Can you work these out from the model? Positions are in its coordinate system, mm. A direction names the side the tool comes from. Give positions to 0.01 mm unless a question says otherwise; leave off trailing zeros. Write each loop counter-clockwise with the first axis right and the second up, starting at its lowest first coordinate (ties: lowest second). Pieces come first, ordered by that corner, then holes. Notation, with made-up numbers: (48.5, 17.25) -> (67.5, 17.25) arc R28 cw to (67.5, 54.25) -> close; hole circle Ø8 at (79.5, 2.5). An arc over 180 degrees is marked (long way). Answer as CSV lines item,"result". Start each with the question number.
1. If we section it at D-D on z = -27: Write out the boundary of the cut face in (x, y).
2. I need wall thicknesses on line 1 (X direction, y = 17, z = -23); line 2 (Y direction, x = 25.5, z = 0); line 3 (Y direction, x = 39, z = 0). Which ranges of each line are inside material? Lowest first, please. Write a range as [from, to].
3. I'm going to push flat-ended pins straight in: P1, Ø21.5, axis at y = 0, z = 0, coming from the -X side; P2, Ø4, axis at y = -1, z = 11.5, coming from the -X side; P3, Ø6, axis at y = -28, z = -3.5, coming from the +X side; P4, Ø12, axis at y = -27, z = 19, coming from the -X side. Where does each tip first touch, or does it pass through?
4. If we mould it in two halves opening along X, with no side actions, what happens to faces 1 (the face through (-45.491, 16, 1)), 2 (the face through (-46.03, -23.81, -22.88)), 3 (the face through (20.707, -9, -4))? For each: pulls with the +X half, pulls with the -X half, needs draft (parallel to the pull), parting line crosses it, or undercut.
5. If we section it at C-C on x = 3: Write out the boundary of the cut face in (y, z).
6. On a 3-axis mill with a long thin cutter (end or side, diameter ignored), from which of +Z, -Z, +X, -X, +Y, -Y can I reach the whole of each face in a straight line? I mean faces 4 (the face through (-16.35, 7.19, 9.37)), 5 (the face through (45.491, -1, 16)), 6 (the face through (49.212, 9.35, -7.47)), 7 (the face through (46.045, -12.053, -11.283)), 8 (the face through (37.91, 7.19, 9.37)). Say none if no direction works.
```python
from build123d import *

# Parameters (mm, degrees)
CUT_EXTRUDE1_DEPTH      = 111.87459973
CUT_EXTRUDE1_DEPTH_BACK = 111.87459973


with BuildPart() as part:
    # Sketch2 → Revolve1 (revolve)
    with BuildSketch(Plane.XY, mode=Mode.PRIVATE) as revolve1_sk:
        Polygon((-52.3875, 11.811), (-52.3875, 12.7), (-46.5836, 12.7), (-46.5836, 36.83), (-45.4914, 36.83), (-45.4914, 12.7), (45.4914, 12.7), (45.4914, 36.83), (46.5836, 36.83), (46.5836, 12.7), (49.2125, 12.7), (49.2125, 11.811), (26.91765, 11.811), (26.91765, 9.36625), (20.70735, 9.36625), (20.70735, 11.811), align=None)
    revolve(revolve1_sk.sketch.rotate(Axis((0, 0, 0), (-1, 0, 0)), 90), axis=Axis((0, 0, 0), (-1, 0, 0)))

    # Sketch3 → Cut-Extrude1 (cut, two sides: drawn at the far end of the back side and taken through both)
    with BuildSketch(Plane.ZY.offset(-45.4914).offset(-CUT_EXTRUDE1_DEPTH_BACK)):
        with BuildLine():
            Line((-18.112952688, -5.32652278), (-29.140106204, -8.569306297))
            ThreePointArc((-29.140106204, -8.569306297), (-30.702095808, -9.883795088), (-30.792130213, -11.923301428))
            ThreePointArc((-30.792130213, -11.923301428), (-22.728159534, -23.953103435), (-10.291997319, -31.375072768))
            ThreePointArc((-10.291997319, -31.375072768), (-8.264508496, -31.180706004), (-7.031658144, -29.559419671))
            Line((-7.031658144, -29.559419671), (-4.327850892, -18.394165222))
            ThreePointArc((-4.327850892, -18.394165222), (-4.548475673, -16.613982469), (-5.890298237, -15.423504358))
            ThreePointArc((-5.890298237, -15.423504358), (-11.349323888, -11.990535738), (-15.076837789, -6.728228762))
            ThreePointArc((-15.076837789, -6.728228762), (-16.331679174, -5.457246069), (-18.112952688, -5.32652278))
        make_face()
    extrude(amount=CUT_EXTRUDE1_DEPTH + CUT_EXTRUDE1_DEPTH_BACK, mode=Mode.SUBTRACT)


solid = part.part
```
Computed values:
1,outline,"(-46.58, -25.05) -> (-45.49, -25.05) -> (-45.49, -19.01) -> (-46.58, -19.01) -> close; (-46.58, -7.94) -> (-45.49, -7.94) -> (-45.49, 25.05) -> (-46.58, 25.05) -> close; (45.49, -25.05) -> (46.58, -25.05) -> (46.58, -19.01) -> (45.49, -19.01) -> close; (45.49, -7.94) -> (46.58, -7.94) -> (46.58, 25.05) -> (45.49, 25.05) -> close"
2,line 1,"x = [-46.58, -45.49], [45.49, 46.58]"
2,line 2,"y = [-12.7, -9.37], [9.37, 12.7]"
2,line 3,"y = [-12.7, -11.81], [11.81, 12.7]"
3,P1,"stops at x = 20.71"
3,P2,"stops at x = -52.39"
3,P3,"stops at x = 46.58"
3,P4,"stops at x = -46.58"
4,face 1,"undercut"
4,face 2,"needs draft"
4,face 3,"pulls with the -X half"
5,outline,"circle Ø25.4 at (0, 0); hole circle Ø23.62 at (0, 0)"
6,face 4,"-X"
6,face 5,"none"
6,face 6,"+Z, -Z, +X, +Y, -Y"
6,face 7,"+X, -X"
6,face 8,"+X"
